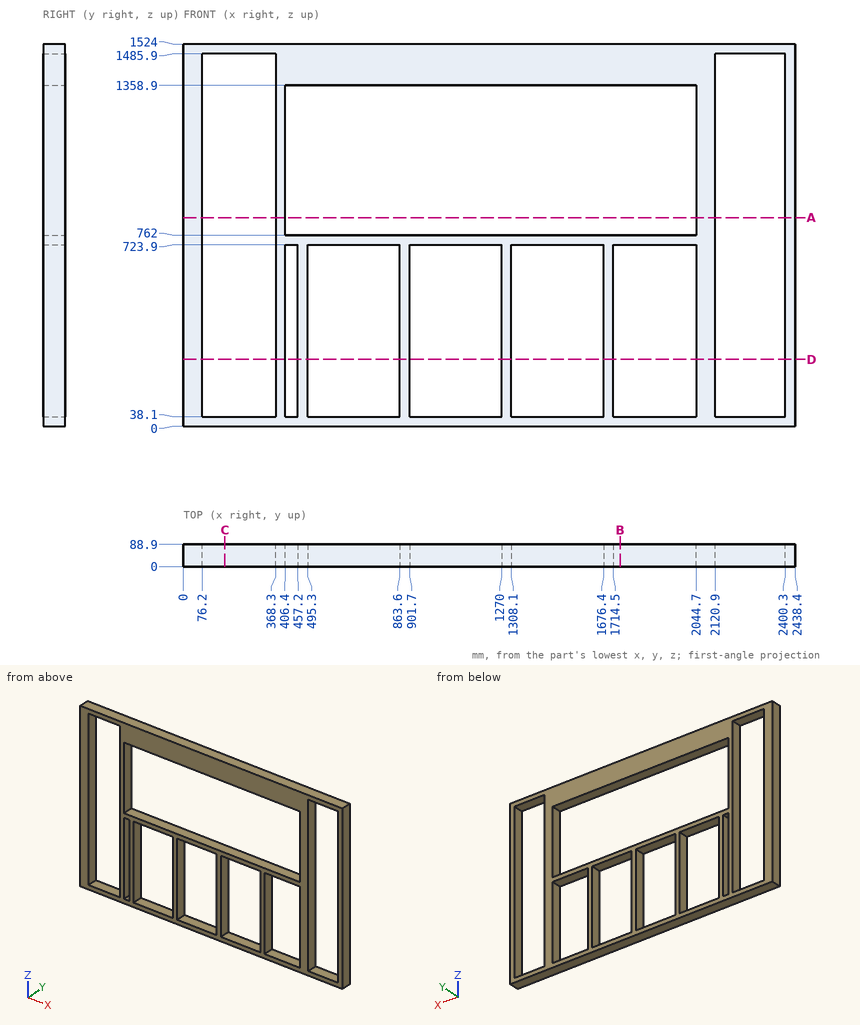
Answer from the drawing. Dimensions are ordinates in mm from the lowest x, y and z of the part. Coordinates: 2 decimals unless noted, no trailing zeros. Loops run counter-clockwise (first coordinate to the right, second up) from the corner with the lowest first, then second, coordinate; pieces in that order, holes last. Notation, with made-up numbers: (-17, 11.25) -> (-2, 11.25) arc R23 ccw to (-2, 26.25) -> close; hole circle Ø6 at (87, 79.25). An arc over 180 degrees is marked (long way). Answer in a Markdown table with one row per item.
Item 1: A cutting plane is placed at B-B on x = 1741. Determine the outline of the cut face in (y, z).
Returned:
| item | result |
|---|---|
| outline | (0, 0) -> (88.9, 0) -> (88.9, 38.1) -> (0, 38.1) -> close; (0, 723.9) -> (88.9, 723.9) -> (88.9, 762) -> (0, 762) -> close; (0, 1358.9) -> (88.9, 1358.9) -> (88.9, 1524) -> (0, 1524) -> close |
Item 2: A cutting plane is placed at C-C on x = 166. Determine the outline of the cut face in (y, z).
Returned:
| item | result |
|---|---|
| outline | (0, 0) -> (88.9, 0) -> (88.9, 38.1) -> (0, 38.1) -> close; (0, 1485.9) -> (88.9, 1485.9) -> (88.9, 1524) -> (0, 1524) -> close |
Item 3: A cutting plane is placed at A-A on z = 831.5. Determine the outline of the cut face in (x, y).
Returned:
| item | result |
|---|---|
| outline | (0, 0) -> (76.2, 0) -> (76.2, 88.9) -> (0, 88.9) -> close; (368.3, 0) -> (406.4, 0) -> (406.4, 88.9) -> (368.3, 88.9) -> close; (2044.7, 0) -> (2120.9, 0) -> (2120.9, 88.9) -> (2044.7, 88.9) -> close; (2400.3, 0) -> (2438.4, 0) -> (2438.4, 88.9) -> (2400.3, 88.9) -> close |
Item 4: Straight lines are drawn through the part: line 1 along Z through (x, y) = (1784, 20.5); line 2 along X through (y, z) = (84, 1273); line 3 along X through (y, z) = (54.5, 1406.5). For each, find the intervals that lie inside material, in ascending order. Write a range as [from, to].
Returned:
| item | result |
|---|---|
| line 1 | z = [0, 38.1], [723.9, 762], [1358.9, 1524] |
| line 2 | x = [0, 76.2], [368.3, 406.4], [2044.7, 2120.9], [2400.3, 2438.4] |
| line 3 | x = [0, 76.2], [368.3, 2120.9], [2400.3, 2438.4] |
Item 5: A cutting plane is placed at D-D on z = 266.5. Give the number of separate pieces and of enclosed holes in the cut face, plus the area to 3 significant figures.
Returned:
| item | result |
|---|---|
| separate pieces | 8 |
| enclosed holes | 0 |
| area | 33,900 mm^2 |
